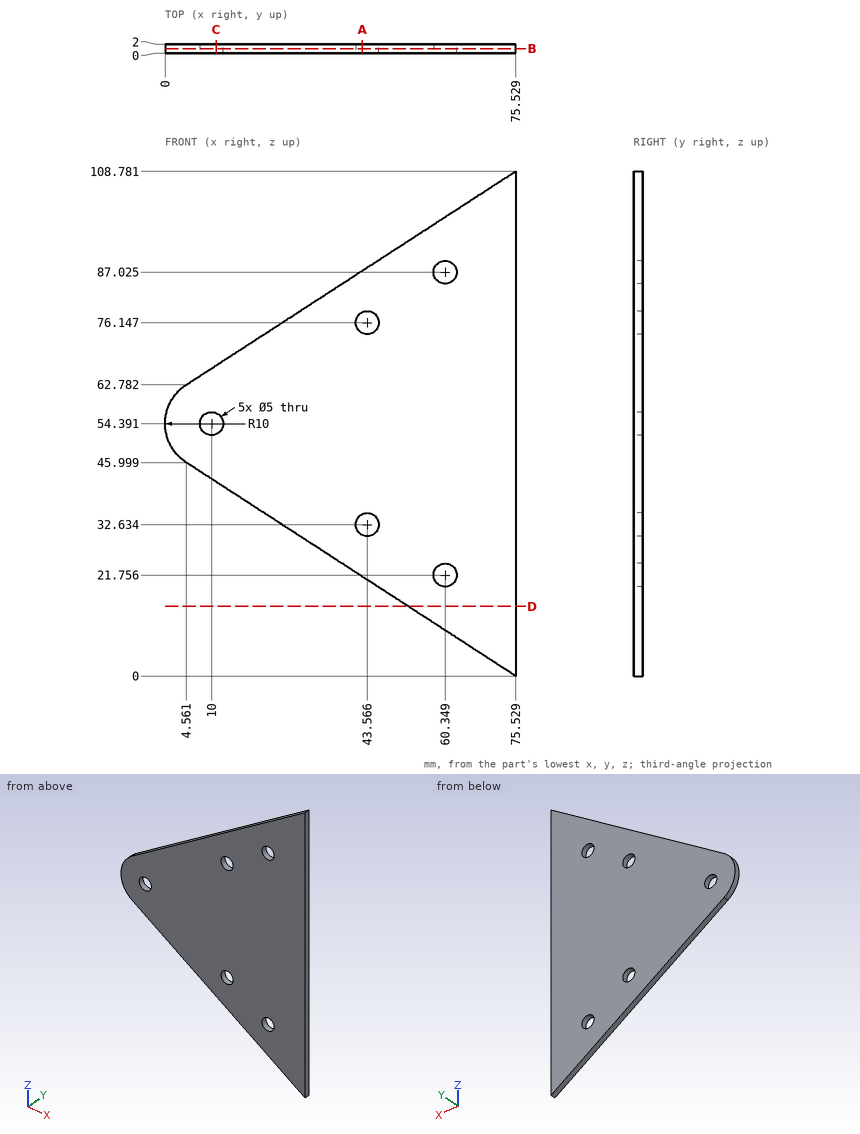
For this review, use the dimensioned drawing (mm, ordinates from the lowest corner) and the shaded views. Give positions to 0.01 mm unless a question says otherwise; leave off trailing zeros. Order: outer loops, then holes, each group sorted by start corner. A loop starts at its lowest first (then second) coordinate and runs counter-clockwise, first axis right, second up. Notation, with made-up numbers: M -29.5,-32 L 11.5,-32 A29 ccw 11.5,7 Z; hole C 14,26 d7. An arc over 180 degrees is marked long. One line per question, with ' | ' between items. Start each with the question number.
1) Wall thickness on L1, parallel to Z at x = 9, y = 1.25; L2, parallel to X at y = 1.2, z = 21 (1 decimal); L3, parallel to X at y = 0.55, z = 54: over which ranges is each line inside the solid? List them lowest first. Write a range as from..to.
2) Consider section A-A, the plane x = 42.5. Give the boundary of the cut face in (y, z) (1 decimal).
3) Consider section D-D, the plane z = 15. Give the boundary of the cut face in (x, y).
4) Consider section C-C, the plane x = 11. Give the boundary of the cut face in (y, z) (1 decimal), then the cut area to 3 significant figures.
5) Clearance check with flat-ended pins moving along their axes: P1, Ø1, axis at x = 66, y = 1.5, coming from the +Z side; P2, Ø1, axis at x = 63, y = 0, coming from the -Z side. State where each tip first meets the part, or that it passes through.
6) Consider section B-B, the plane y = 1. Give the boundary of the cut face in (x, z) (1 decimal), then the cut area to 3 significant figures.
Found:
1) L1: z = 43.12..52.1, 56.68..65.66 | L2: x = 43.1..58, 62.7..75.5 | L3: x = 0.01..7.53, 12.47..75.53
2) outline: M 0,21.4 L 2,21.4 L 2,30.4 L 0,30.4 Z; M 0,34.9 L 2,34.9 L 2,73.9 L 0,73.9 Z; M 0,78.4 L 2,78.4 L 2,87.4 L 0,87.4 Z
3) outline: M 52.39,0 L 75.53,0 L 75.53,2 L 52.39,2 Z
4) outline: M 0,41.8 L 2,41.8 L 2,52.1 L 0,52.1 Z; M 0,56.7 L 2,56.7 L 2,67 L 0,67 Z | area: 41.1 mm²
5) P1: stops at z = 102.93 | P2: stops at z = 7.8
6) outline: M 4.6,46 L 75.5,0 L 75.5,108.8 L 4.6,62.8 A10 ccw Z; hole C 10,54.4 d5; hole C 43.6,32.6 d5; hole C 43.6,76.1 d5; hole C 60.3,21.8 d5; hole C 60.3,87 d5 | area: 4,410 mm²
